For this review, take the finished solid that the model builds, in its own axes (mm). A direction names the side the tool comes from. Give positions to 0.01 mm unless a question says otherwise; leave off trailing zeros. Order: outer loops, then holes, each group sorted by start corner. A loop starts at its lowest first (then second) coordinate and runs counter-clockwise, first axis right, second up.
Item 1: For probe 1 along X at (y, z) = (65.5, 0.7); probe 2 along Y at (x, z) = (21.5, 1.3); probe 3 along Y at (x, z) = (17.75, 0.7), list the stretches that pass through material, from the lowest coordinate up.
Item 2: Consider section A-A (y = 12.7). Give the boundary of the cut face in (x, z), plus the area to 3 significant figures.
Item 3: Consider section C-C (y = 35.26). Give the boundary of the cut face in (x, z).
Item 4: Consider section D-D (z = 2.35). Give the number of separate pieces and of enclosed holes in the cut face, plus the area to 3 significant figures.
Item 5: For P1, Ø4, axis at x = 12.7, y = 12.7, coming from the +Z side, flat-tipped, find the tip position at first contact; note if it passes through.
Item 6: Consider section B-B (x = 12.7). Give the boundary of the cut face in (y, z), plus the area to 3 significant figures.
Item 7: The part is to be moulded in two halves that separate along X. For faces 1 (the cylindrical face through (0.91, 0.95, 2.41)), 2 (the cylindrical face through (10.403, 5.687, 2.348)), 3 (the flat face through (13, 0, 2)), 4 (the flat face through (25.4, 44, 2)), say which applies: released by +X, released by -X, zero draft, split by the parting line, or undercut.
Item 8: Machinability: for faces 5 (the flat face through (2.7, 59, 2)), 6 (the flat face through (13, 35, 4.762)), which of the approach directions +Z, -Z, +X, -X, +Y, -Y give a long, thin tool a straight path to every point of the face, cutting with its end or side? Answer none if there is none.
```python
from build123d import *

# Parameters (mm, degrees)
SKETCH1_W           = 25.4
SKETCH1_H           = 88.9
SKETCH1_R           = 2
SKETCH1_R_2         = 10
SKETCH1_W_2         = 20
SKETCH1_H_2         = 40.9
SKETCH1_R_3         = 1.5
SKETCH1_R_4         = 0.75
BOSS_EXTRUDE1_DEPTH = 4.7625
FILLET1_R           = 3.175
SKETCH2_R           = 2.2
CUT_EXTRUDE1_DEPTH  = 93.57997303


with BuildPart() as part:
    # Sketch1 → Boss-Extrude1 (new body)
    # profile 1 of 2: a face of its own
    with BuildSketch(Plane.XY):
        with Locations((12.7, 44.45)):
            Rectangle(SKETCH1_W, SKETCH1_H)
        with Locations(Location((17.7, 35.26, 0), (0, 0, 180))):
            Circle(SKETCH1_R, mode=Mode.SUBTRACT)
        with Locations(Location((7.7, 35.26, 0), (0, 0, 180))):
            Circle(SKETCH1_R, mode=Mode.SUBTRACT)
        with Locations(Location((17.7, 83.86, 0), (0, 0, 180))):
            Circle(SKETCH1_R, mode=Mode.SUBTRACT)
        with Locations(Location((7.7, 83.86, 0), (0, 0, 180))):
            Circle(SKETCH1_R, mode=Mode.SUBTRACT)
        with Locations((12.7, 12.7)):
            Circle(SKETCH1_R_2, mode=Mode.SUBTRACT)
        with Locations((12.7, 59.56)):
            Rectangle(SKETCH1_W_2, SKETCH1_H_2, mode=Mode.SUBTRACT)
    # profile 2 of 2: a face of its own
    with BuildSketch(Plane.XY):
        with Locations((12.7, 12.7)):
            Circle(SKETCH1_R_2)
        with Locations(Location((12.7, 12.7, 0), (0, 0, 180))):
            Circle(SKETCH1_R_3, mode=Mode.SUBTRACT)
        with Locations(Location((10.092137103, 19.855351222, 0), (0, 0, 180))):
            Circle(SKETCH1_R_4, mode=Mode.SUBTRACT)
        with Locations(Location((7.906074869, 17.80081188, 0), (0, 0, 180))):
            Circle(SKETCH1_R_4, mode=Mode.SUBTRACT)
        with Locations(Location((5.720012634, 15.746272538, 0), (0, 0, 180))):
            Circle(SKETCH1_R_4, mode=Mode.SUBTRACT)
        with Locations(Location((5.544648778, 10.092137103, 0), (0, 0, 180))):
            Circle(SKETCH1_R_4, mode=Mode.SUBTRACT)
        with Locations(Location((7.59918812, 7.906074869, 0), (0, 0, 180))):
            Circle(SKETCH1_R_4, mode=Mode.SUBTRACT)
        with Locations(Location((9.653727462, 5.720012634, 0), (0, 0, 180))):
            Circle(SKETCH1_R_4, mode=Mode.SUBTRACT)
        with Locations(Location((15.307862897, 5.544648778, 0), (0, 0, 180))):
            Circle(SKETCH1_R_4, mode=Mode.SUBTRACT)
        with Locations(Location((17.493925131, 7.59918812, 0), (0, 0, 180))):
            Circle(SKETCH1_R_4, mode=Mode.SUBTRACT)
        with Locations(Location((19.679987366, 9.653727462, 0), (0, 0, 180))):
            Circle(SKETCH1_R_4, mode=Mode.SUBTRACT)
        with Locations(Location((19.855351222, 15.307862897, 0), (0, 0, 180))):
            Circle(SKETCH1_R_4, mode=Mode.SUBTRACT)
        with Locations(Location((17.80081188, 17.493925131, 0), (0, 0, 180))):
            Circle(SKETCH1_R_4, mode=Mode.SUBTRACT)
        with Locations(Location((15.746272538, 19.679987366, 0), (0, 0, 180))):
            Circle(SKETCH1_R_4, mode=Mode.SUBTRACT)
    extrude(amount=BOSS_EXTRUDE1_DEPTH)

    # Fillet1
    fillet1_edges = [part.edges().sort_by_distance(p)[0] for p in [
        (0, 0, 2.38125),
        (0, 88.9, 2.38125),
        (25.4, 88.9, 2.38125),
        (25.4, 0, 2.38125),
    ]]
    fillet(fillet1_edges, radius=FILLET1_R)

    # Sketch2 → Cut-Extrude1 (cut, through all)
    with BuildSketch(Plane.XY.offset(4.7625)):
        with Locations((12.7, 12.7)):
            Circle(SKETCH2_R)
    extrude(amount=-CUT_EXTRUDE1_DEPTH, mode=Mode.SUBTRACT)


solid = part.part
```
Resolved:
1. probe 1: x = 0 to 2.7, 22.7 to 25.4
1. probe 2: y = 0 to 39.11, 80.01 to 88.9
1. probe 3: y = 0 to 6.89, 8.3 to 16.75, 18.24 to 33.26, 37.26 to 39.11, 80.01 to 81.86, 85.86 to 88.9
2. outline: (0, 0) - (10.5, 0) - (10.5, 4.76) - (0, 4.76) - close; (14.9, 0) - (25.4, 0) - (25.4, 4.76) - (14.9, 4.76) - close
2. area: 100 mm2
3. outline: (0, 0) - (5.7, 0) - (5.7, 4.76) - (0, 4.76) - close; (9.7, 0) - (15.7, 0) - (15.7, 4.76) - (9.7, 4.76) - close; (19.7, 0) - (25.4, 0) - (25.4, 4.76) - (19.7, 4.76) - close
4. separate pieces: 1
4. enclosed holes: 18
4. area: 1,340 mm2
5. P1: passes through
6. outline: (0, 0) - (10.5, 0) - (10.5, 4.76) - (0, 4.76) - close; (14.9, 0) - (39.11, 0) - (39.11, 4.76) - (14.9, 4.76) - close; (80.01, 0) - (88.9, 0) - (88.9, 4.76) - (80.01, 4.76) - close
6. area: 208 mm2
7. face 1: released by -X
7. face 2: undercut
7. face 3: zero draft
7. face 4: released by +X
8. face 5: +Z, -Z
8. face 6: +Z, +X, -X, +Y, -Y
